from build123d import *

# Parameters (mm, degrees)
F0_R        = 10
F1_DEPTH    = 120
F2_T1_DEPTH = 388.0868278764
F3_R        = 83.3946881549
F4_R        = 360.5996262689
F5_W        = 10.426518289
F5_H        = 107.3879271778
F5_W_2      = 9.573481711
F6_DEPTH    = 80
F7_T1_DEPTH = 238.837194796
F7_T3_DEPTH = 237.984158218
F9_D        = 20


# Not quite as in the source:
# - a fillet or chamfer that OpenCascade refuses, or shapes differently, is made with other operations: its cross-section is extruded or revolved along the edge and cut away or added


with BuildPart() as f1:
    # F0 (on Front) → F1 (new body)
    with BuildSketch(Plane.XZ):
        Polygon((240.6433847223, 159.6522270207), (-900.6182220181, 159.6522270207), (-900.6182220181, 59.6522270207), (200.0234600665, 59.6522270207), align=None)
        with Locations((-816.3304328918, 103.5160794854)):
            Circle(F0_R, mode=Mode.SUBTRACT)
        Polygon((786.7558863362, -272.8294734313), (240.6433847223, 159.6522270207), (200.0234600665, 59.6522270207), (720.0863678131, -357.0158274528), align=None)
        with Locations((710.3598117828, -279.6283066273)):
            Circle(F0_R, mode=Mode.SUBTRACT)
    extrude(amount=F1_DEPTH)

    # F2: fillet of radius 53.6173655753 on 2 edges, made by hand

    # F2_s2 → F2_t1 (cut)
    with BuildSketch(Plane.XZ.offset(-134.0434139382)):
        with BuildLine():
            ThreePointArc((-847.0008564428, 159.6522270207), (-884.9140592305, 143.9480642331), (-900.6182220181, 106.0348614454))
            Line((-900.6182220181, 106.0348614454), (-900.6182220181, 159.6522270207))
            Line((-900.6182220181, 159.6522270207), (-847.0008564428, 159.6522270207))
        make_face()
        with BuildLine():
            ThreePointArc((-900.6182220181, 113.269592596), (-884.9140592305, 75.3563898084), (-847.0008564428, 59.6522270207))
            Line((-847.0008564428, 59.6522270207), (-900.6182220181, 59.6522270207))
            Line((-900.6182220181, 59.6522270207), (-900.6182220181, 113.269592596))
        make_face()
    extrude(amount=F2_T1_DEPTH, mode=Mode.SUBTRACT)

    # F3
    f3_edges = [f1.edges().sort_by_distance(p)[0] for p in [
        (240.643385, -60, 159.652227),
    ]]
    fillet(f3_edges, radius=F3_R)

    # F4
    f4_edges = [f1.edges().sort_by_distance(p)[0] for p in [
        (200.02346, -60, 59.652227),
    ]]
    fillet(f4_edges, radius=F4_R)

    # F5 (on face) → F6 (join)
    with BuildSketch(Plane(origin=(616.3029320724, 0, -488.0674572886), x_dir=(0, 1, 0), z_dir=(0.7839461682, 0, -0.6208288052))):
        with Locations((-114.7867408555, 220.8631330454)):
            Rectangle(F5_W, F5_H)
        with Locations((-4.7867408555, 220.8631330454)):
            Rectangle(F5_W_2, F5_H)
    extrude(amount=F6_DEPTH)

    # F7: fillet of radius 45.6821353014 on 5 edges, made by hand

    # F7_s2 → F7_t1 (cut)
    with BuildSketch(Plane.XZ.offset(-4.6318565425)):
        with BuildLine():
            ThreePointArc((811.1628467471, -370.8697969446), (780.6195529663, -387.886260073), (746.9897263442, -378.3213463908))
            Line((746.9897263442, -378.3213463908), (782.8020612687, -406.6821318691))
            Line((782.8020612687, -406.6821318691), (811.1628467471, -370.8697969446))
        make_face()
        with BuildLine():
            ThreePointArc((821.1107943135, -358.3081127721), (830.6757079957, -324.6782861501), (813.6592448673, -294.1349923693))
            Line((813.6592448673, -294.1349923693), (849.4715797918, -322.4957778476))
            Line((849.4715797918, -322.4957778476), (821.1107943135, -358.3081127721))
        make_face()
    extrude(amount=F7_T1_DEPTH, mode=Mode.SUBTRACT)

    # F7_s4 → F7_t3 (cut)
    with BuildSketch(Plane.XZ.offset(-114.2053382535)):
        with BuildLine():
            ThreePointArc((811.1628467471, -370.8697969446), (780.6195529663, -387.886260073), (746.9897263442, -378.3213463908))
            Line((746.9897263442, -378.3213463908), (782.8020612687, -406.6821318691))
            Line((782.8020612687, -406.6821318691), (811.1628467471, -370.8697969446))
        make_face()
        with BuildLine():
            ThreePointArc((813.6592448673, -294.1349923693), (830.6757079957, -324.6782861501), (821.1107943135, -358.3081127721))
            Line((821.1107943135, -358.3081127721), (849.4715797918, -322.4957778476))
            Line((849.4715797918, -322.4957778476), (813.6592448673, -294.1349923693))
        make_face()
    extrude(amount=F7_T3_DEPTH, mode=Mode.SUBTRACT)

    # F9 (through all)
    with Locations(Plane(origin=(0, 0, 0), x_dir=(-1, 0, 0), z_dir=(0, 1, 0))):
        with Locations((-781.1415195465, -335.5341851711)):
            Hole(F9_D / 2)


solid = f1.part
Design review of the part built by this model. Coordinates are the model's own, in mm. A direction names the side the tool comes from. Give positions to 0.01 mm unless a question says otherwise; leave off trailing zeros. Order: outer loops, then holes, each group sorted by start corner. A loop starts at its lowest first (then second) coordinate and runs counter-clockwise, first axis right, second up.
1. Tool access review of faces 5 (the flat face through (791, -109.573, -331)), 6 (the flat face through (-393, -59, 59.652)), 7 (the flat face through (-310, -59, 159.652)): name each direction out of +Z, -Z, +X, -X, +Y, -Y from which nothing blocks a thin tool from reaching the whole face with its end or side.
Solution:
face 5: -Z, +X
face 6: -Z, -X, +Y, -Y
face 7: +Z, +X, -X, +Y, -Y
2. Add section C-C, the plane z = -45.5. State the section outline as (x, y) points.
Solution:
outline: (331.27, -120) - (499.7, -120) - (499.7, 0) - (331.27, 0) - close
3. Mouldability with a two-part tool opening along Y and no side actions: class faces 1 (the flat face through (25, 0, 90)), 2 (the flat face through (752.954, -58.873, -315.512)), 3 (the flat face through (36, -120, 84)), 4 (the cylindrical face through (-883.2, -59.16, 145.59)) as +Y half, -Y half, draft (parallel to the pull), parting line (faces both ways), or undercut.
Solution:
face 1: +Y half
face 2: undercut
face 3: -Y half
face 4: draft
4. For pin 1 Ø12 at (y, z) = (-88.5, -25) entering from +X; pin 2 Ø23 at (x, z) = (710.36, -279.63) entering from -Y; pin 3 Ø4 at (x, y) = (212, -97.5) entering from -Z; pin 4 Ø4 at (y, z) = (-33.5, -118.5) entering from +X, all flat-tipped, find the tip position at first contact; note any pin that passes through.
Solution:
pin 1: stops at x = 481.39
pin 2: stops at y = -120
pin 3: stops at z = 31.11
pin 4: stops at x = 594.4
5. To check wall thickness, follow L1, parallel to Z at x = -399.5, y = -56; L2, parallel to X at y = -33, z = -281.5; L3, parallel to Z at x = 112, y = -62.5. State the ranges of each line that lie inside material, in increasing order.
Solution:
L1: z = 59.65 to 159.65
L2: x = 625.83 to 700.54, 720.18 to 779.89
L3: z = 57.58 to 159.65
6. Add section B-B, the plane x = 505. State the section outline as (y, z) points.
Solution:
outline: (-120, -184.69) - (0, -184.69) - (0, -49.7) - (-120, -49.7) - close
7. Add section A-A, the plane y = -69. State the section outline as (x, z) points.
Solution:
outline: (-900.5, 109.65) arc R53.62 ccw to (-847, 59.65) - (73.39, 59.65) arc R360.6 cw to (298.85, -19.53) - (720.09, -357.02) - (786.76, -272.83) - (263.4, 141.63) arc R83.39 ccw to (211.62, 159.65) - (-847, 159.65) arc R53.62 ccw to start; hole circle Ø20 at (-816.33, 103.52); hole circle Ø20 at (710.36, -279.63)
